```python
from build123d import *

# Parameters (mm, degrees)
F0_W     = 30
F0_H     = 30
F0_R     = 4.25
F1_DEPTH = 12
F2_SIZE  = 0.5


with BuildPart() as f1:
    # F0 (on Top) → F1 (new body)
    with BuildSketch(Plane.XY):
        Rectangle(F0_W, F0_H)
        Circle(F0_R, mode=Mode.SUBTRACT)
    extrude(amount=F1_DEPTH)

    # F2
    f2_edges = [f1.edges().sort_by_distance(p)[0] for p in [
        (4.25, 0, 6),
        (-4.25, 0, 0),
        (-4.25, 0, 12),
    ]]
    chamfer(f2_edges, length=F2_SIZE)


solid = f1.part
```
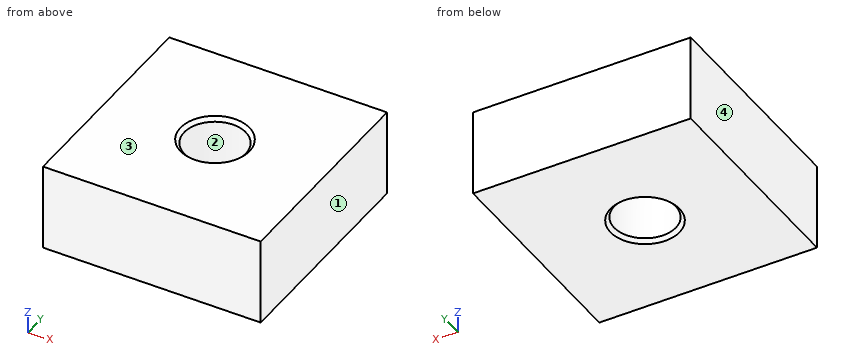
Verification items for the finished model (mm, model axes). Face numbers are marked on the shaded views. Give positions to 0.01 mm unless a question says otherwise; leave off trailing zeros. Write each loop counter-clockwise with the first axis right and the second up, starting at its lowest first coordinate (ties: lowest second). Pieces come first, ordered by that corner, then holes. Notation, with made-up numbers: M -38,-1 L -15,-1 A18 ccw -15,25 Z; hole C 45,67 d5. An arc over 180 degrees is marked long. One line per question, with ' | ' between items.
1) Section check A-A on x = 0. Enter the section's corners in (y, z), plus the area to 4 significant figures.
Result:
outline: M -15,0 L -4.75,0 L -4.25,0.5 L -4.25,11.5 L -4.75,12 L -15,12 Z; M 4.25,0.5 L 4.75,0 L 15,0 L 15,12 L 4.75,12 L 4.25,11.5 Z | area: 257.5 mm2
2) Section check C-C on z = 8.75. Enter the section's corners in (x, y).
Result:
outline: M -15,-15 L 15,-15 L 15,15 L -15,15 Z; hole C 0,0 d8.5
3) Mould release check, pull along X, two halves, no side actions. Record for the marked faces 1, 2, 3 and 4: released by +X, released by -X, zero draft, split by the parting line, or undercut.
Result:
face 1: released by +X | face 2: undercut | face 3: zero draft | face 4: released by -X
4) Thickness scan on line 1 along Y through (x, z) = (0, 9.25); line 2 along X through (y, z) = (-1.75, 1.5); line 3 along Y through (x, z) = (-1.5, 10). Record the ranges inside material, lowest first. Write a range as [from, to].
Result:
line 1: y = [-15, -4.25], [4.25, 15] | line 2: x = [-15, -3.87], [3.87, 15] | line 3: y = [-15, -3.98], [3.98, 15]
